```python
from build123d import *

# Parameters (mm, degrees)
PAD_DEPTH = 152.4


with BuildPart() as part:
    # Sketch → Pad (new body, symmetric)
    with BuildSketch(Plane.YZ):
        Polygon((-88.9, 100.584), (-88.9, -1.016), (88.9, -1.016), (88.9, 100.584), (87.884, 100.584), (87.884, 0), (-87.884, 0), (-87.884, 100.584), align=None)
    extrude(amount=PAD_DEPTH, both=True)


solid = part.part
```
CAD build for the part. Positions are in the model's coordinates, mm. A direction names the side the tool comes from. Round coordinates to 2 decimals unless told otherwise and drop trailing zeros. Write each loop counter-clockwise with the first axis right and the second up, starting at its lowest first coordinate (ties: lowest second). Pieces come first, ordered by that corner, then holes. Notation, with made-up numbers: (-1, 62) - (9, 62) arc R26 ccw to (9, 86) - close; hole circle Ø6 at (14, 1). An arc over 180 degrees is marked (long way). Write item = value, one per line. Start each with the question number.
Q1. Drop a flat-ended pin along its axis: pin 1 (8 mm diameter, centred on x = 54.5, y = -58, fed in from +Z). Give the stop position or say it passes through.
Q2. Band-saw the part on C-C (y = -70.5). Give the cut face in (x, z).
Q3. Mould opens along Y. For faces 1 (the flat face through (2, 87.884, 51)), 2 (the flat face through (2, -1, -1.016)), 3 (the flat face through (2, -88.9, 50)) say: pulls with the +Y half, pulls with the -Y half, needs draft (parallel to the pull), parting line crosses it, or undercut.
Q4. Which spindle directions (+Z, -Z, +X, -X, +Y, -Y) get a long thin tool onto all of the face, cutting with end or side? Do faces 4 (the flat face through (2, 88.9, 49)), 5 (the flat face through (2, 1, 0)). Say none if no direction does.
Q5. Band-saw the part on A-A (z = 54.5). Give the cut face in (x, y), then the cut area to 3 significant figures.
Q6. Band-saw the part on B-B (x = 118). Give the cut face in (y, z), then the cut area to 3 significant figures.
Q7. Probe L1, parallel to Y at x = 109, z = 40; L2, parallel to Z at x = -99, y = 56. List the from-to ranges inside material, lowest first. Write a range as from..to.
Answers below:
q1.pin_1 = 0
q2.outline = (-152.4, -1.02) - (152.4, -1.02) - (152.4, 0) - (-152.4, 0) - close
q3.face_1 = undercut
q3.face_2 = needs draft
q3.face_3 = pulls with the -Y half
q4.face_4 = +Z, -Z, +X, -X, +Y
q4.face_5 = +Z, +X, -X
q5.outline = (-152.4, -88.9) - (152.4, -88.9) - (152.4, -87.88) - (-152.4, -87.88) - close; (-152.4, 87.88) - (152.4, 87.88) - (152.4, 88.9) - (-152.4, 88.9) - close
q5.area = 619 mm2
q6.outline = (-88.9, -1.02) - (88.9, -1.02) - (88.9, 100.58) - (87.88, 100.58) - (87.88, 0) - (-87.88, 0) - (-87.88, 100.58) - (-88.9, 100.58) - close
q6.area = 385 mm2
q7.L1 = -88.9..-87.88, 87.88..88.9
q7.L2 = -1.02..0
